Source: three-view drawing plus pictorial views. Frame: mm from the lowest corner of the part. A direction names the side the tool comes from. Round coordinates to 2 decimals unless told otherwise and drop trailing zeros. Loops run counter-clockwise (first coordinate to the right, second up) from the corner with the lowest first, then second, coordinate; pieces in that order, holes last. Notation, with made-up numbers: (41, 32) -> (47, 32) arc R16 cw to (47, 43) -> close; hole circle Ø8 at (23, 70.5). An arc over 180 degrees is marked (long way). One line per question, with ' | ' between items. Start each with the question number.
Q1. Material intervals for L1, parallel to Z at x = 35.5, y = 0.95; L2, parallel to X at y = 1.05, z = 4.5 (1 decimal), sorted ascending.
Q2. Cut plane A-A on x = 5. Return loops of the section in (y, z).
Q3. Cut plane D-D on z = 16. Return loops of the section in (x, y), and give its area (3 significant figures).
Q4. Cut plane C-C on x = 31. Return loops of the section in (y, z).
Q5. Cut plane B-B on z = 35.5. Return loops of the section in (x, y).
Q6. Access query for the marked faces 1 and 2. Directions: +Z, -Z, +X, -X, +Y, -Y. A direction counts if a zero-diameter tool reaches every point of the face in a straight line with its end or side. Return the directions, or none.
Q7. Contact query for flat-ended pins moving along their axis: P1, Ø0.8, axis at y = 2.5, z = 22.5, coming from the +X side; P2, Ø0.8, axis at x = 15.5, y = 2.5, coming from the +Z side; P3, Ø3, axis at x = 15.5, z = 21.5, coming from the +Y side; P4, Ø2.5, axis at x = 5, z = 5, coming from the -Y side. Output: stop coordinate, or through.
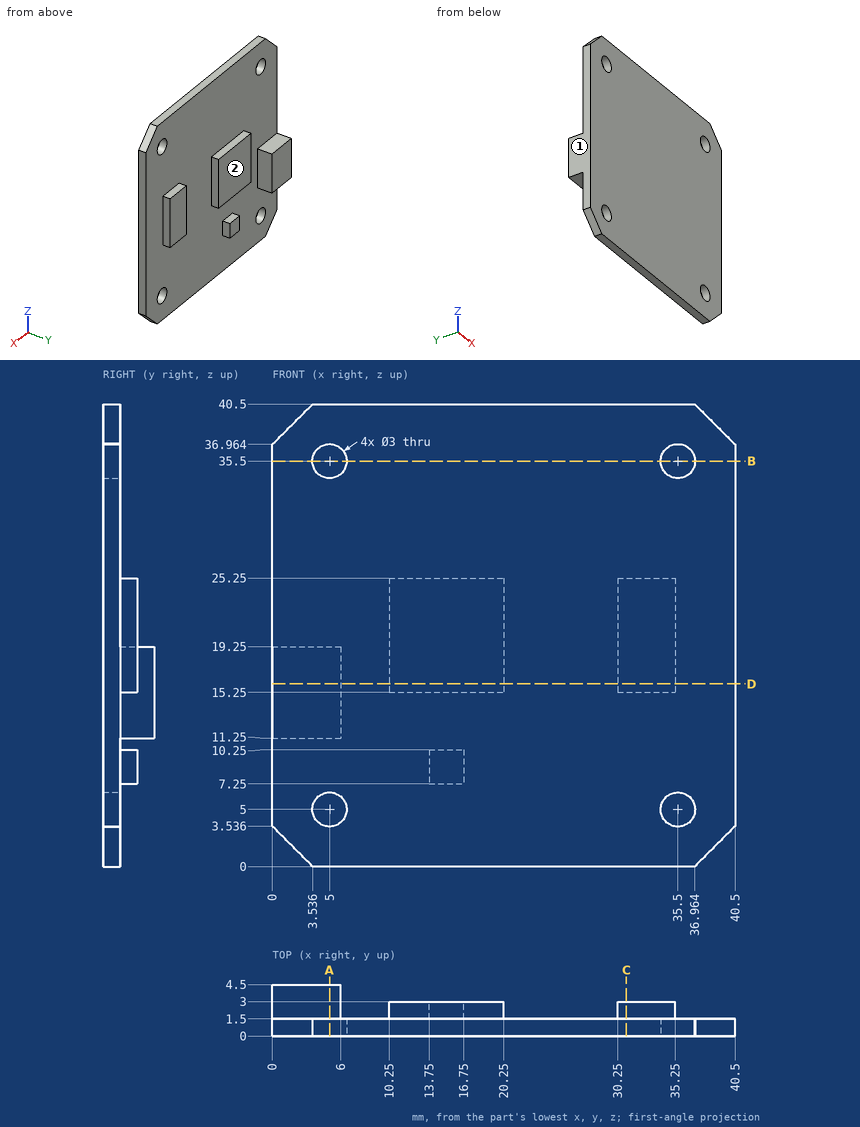
Results:
1) L1: 0 to 3.5, 6.5 to 34, 37 to 40.5 | L2: 0 to 3.6, 6.4 to 34.1, 36.9 to 40.5
2) outline: (0, 0) -> (1.5, 0) -> (1.5, 3.5) -> (0, 3.5) -> close; (0, 6.5) -> (1.5, 6.5) -> (1.5, 11.25) -> (4.5, 11.25) -> (4.5, 19.25) -> (1.5, 19.25) -> (1.5, 34) -> (0, 34) -> close; (0, 37) -> (1.5, 37) -> (1.5, 40.5) -> (0, 40.5) -> close
3) outline: (0, 0) -> (40.5, 0) -> (40.5, 1.5) -> (35.25, 1.5) -> (35.25, 3) -> (30.25, 3) -> (30.25, 1.5) -> (20.25, 1.5) -> (20.25, 3) -> (10.25, 3) -> (10.25, 1.5) -> (6, 1.5) -> (6, 4.5) -> (0, 4.5) -> close | area: 101 mm^2
4) outline: (0, 0) -> (1.5, 0) -> (1.5, 15.25) -> (3, 15.25) -> (3, 25.25) -> (1.5, 25.25) -> (1.5, 40.5) -> (0, 40.5) -> close
5) outline: (0, 0) -> (3.5, 0) -> (3.5, 1.5) -> (0, 1.5) -> close; (6.5, 0) -> (34, 0) -> (34, 1.5) -> (6.5, 1.5) -> close; (37, 0) -> (40.5, 0) -> (40.5, 1.5) -> (37, 1.5) -> close
6) face 1: +Z, -Z, -X, +Y, -Y | face 2: +Z, -Z, +X, +Y
7) P1: x = 35.25 | P2: z = 25.25 | P3: y = 3 | P4: through
